```python
from build123d import *

# Parameters (mm, degrees)
SKETCH_1_W                   = 417.3
SKETCH_1_H                   = 60
EXTRUDE_1_DEPTH              = 23.5
SKETCH_2_W                   = 400
SKETCH_2_H                   = 45
CUT_EXTRUDE_1_DEPTH          = 10
SKETCH_3_W                   = 17.3
SKETCH_3_H                   = 60
EXTRUDE_2_DEPTH              = 19
HOLE_WIZARD_M3_1_D           = 2.5
HOLE_WIZARD_M3_1_DEPTH       = 7.5
HOLE_WIZARD_M3_1_CSINK_D     = 3.05
HOLE_WIZARD_M3_1_CSINK_ANGLE = 90
HOLE_WIZARD_M3_1_TIP         = 0.751075774
FILLET_1_R                   = 5
FILLET_2_R                   = 3
SKETCH_6_R                   = 13
CUT_EXTRUDE_2_DEPTH          = 20
HOLE_WIZARD_M4_1_D           = 3.3
HOLE_WIZARD_M4_1_DEPTH       = 10.1
HOLE_WIZARD_M4_1_CSINK_D     = 4.05
HOLE_WIZARD_M4_1_CSINK_ANGLE = 90
HOLE_WIZARD_M4_1_TIP         = 0.991420021
SKETCH_9_R                   = 2.25
CUT_EXTRUDE_3_DEPTH          = 15


with BuildPart() as part:
    # 草图1 → 凸台-拉伸1 (new body)
    with BuildSketch(Plane.XY):
        with Locations((208.65, -30)):
            Rectangle(SKETCH_1_W, SKETCH_1_H)
    extrude(amount=EXTRUDE_1_DEPTH)

    # 草图2 → 切除-拉伸1 (cut)
    with BuildSketch(Plane.XY.offset(23.5)):
        with Locations((217.3, -30)):
            Rectangle(SKETCH_2_W, SKETCH_2_H)
    extrude(amount=-CUT_EXTRUDE_1_DEPTH, mode=Mode.SUBTRACT)

    # 草图3 → 凸台-拉伸2 (add)
    with BuildSketch(Plane.XY.offset(23.5)):
        with Locations((8.65, -30)):
            Rectangle(SKETCH_3_W, SKETCH_3_H)
    extrude(amount=EXTRUDE_2_DEPTH)

    # M3 螺纹孔1
    with Locations(Plane(origin=(417.3, 0, 0), x_dir=(0, 0, -1), z_dir=(1, 0, 0))):
        with Locations((-4.75, -4), (-18.75, -4), (-18.75, -56), (-4.75, -56)):
            CounterSinkHole(HOLE_WIZARD_M3_1_D / 2, HOLE_WIZARD_M3_1_CSINK_D / 2, depth=HOLE_WIZARD_M3_1_DEPTH, counter_sink_angle=HOLE_WIZARD_M3_1_CSINK_ANGLE)
            with Locations((0, 0, -(HOLE_WIZARD_M3_1_DEPTH + HOLE_WIZARD_M3_1_TIP / 2))):  # 118° drill point
                Cone(0, HOLE_WIZARD_M3_1_D / 2, HOLE_WIZARD_M3_1_TIP, mode=Mode.SUBTRACT)

    # 圆角1
    fillet_1_edges = [part.edges().sort_by_distance(p)[0] for p in [
        (217.3, 0, 23.5),
        (217.3, -60, 23.5),
        (208.65, 0, 0),
        (208.65, -60, 0),
    ]]
    fillet(fillet_1_edges, radius=FILLET_1_R)

    # 圆角2
    fillet_2_edges = [part.edges().sort_by_distance(p)[0] for p in [
        (8.65, -60, 42.5),
        (8.65, 0, 42.5),
    ]]
    fillet(fillet_2_edges, radius=FILLET_2_R)

    # 草图6 → 切除-拉伸2 (cut)
    with BuildSketch(Plane.ZY):
        with Locations(Location((21.3, -30, 0), (0, 0, 270))):
            Circle(SKETCH_6_R)
    extrude(amount=-CUT_EXTRUDE_2_DEPTH, mode=Mode.SUBTRACT)

    # M4 螺纹孔1
    with Locations(Plane.ZY):
        with Locations((9.25, -11), (33.25, -11), (33.25, -49), (9.25, -49)):
            CounterSinkHole(HOLE_WIZARD_M4_1_D / 2, HOLE_WIZARD_M4_1_CSINK_D / 2, depth=HOLE_WIZARD_M4_1_DEPTH, counter_sink_angle=HOLE_WIZARD_M4_1_CSINK_ANGLE)
            with Locations((0, 0, -(HOLE_WIZARD_M4_1_DEPTH + HOLE_WIZARD_M4_1_TIP / 2))):  # 118° drill point
                Cone(0, HOLE_WIZARD_M4_1_D / 2, HOLE_WIZARD_M4_1_TIP, mode=Mode.SUBTRACT)

    # 草图9 → 切除-拉伸3 (cut)
    with BuildSketch(Plane(origin=(0, 0, 0), x_dir=(-1, 0, 0), z_dir=(0, 0, -1))):
        with Locations((-367.3, -15)):
            Circle(SKETCH_9_R)
        with Locations((-267.3, -15)):
            Circle(SKETCH_9_R)
        with Locations((-167.3, -15)):
            Circle(SKETCH_9_R)
        with Locations((-67.3, -15)):
            Circle(SKETCH_9_R)
        with Locations((-267.3, -45)):
            Circle(SKETCH_9_R)
        with Locations((-167.3, -45)):
            Circle(SKETCH_9_R)
        with Locations((-67.3, -45)):
            Circle(SKETCH_9_R)
        with Locations((-367.3, -45)):
            Circle(SKETCH_9_R)
    extrude(amount=-CUT_EXTRUDE_3_DEPTH, mode=Mode.SUBTRACT)


solid = part.part
```
Work out the finished part from the listing and answer in its coordinate system (mm). A direction names the side the tool comes from. Coordinates: 2 decimals unless noted, no trailing zeros. Write each loop counter-clockwise with the first axis right and the second up, starting at its lowest first coordinate (ties: lowest second). Pieces come first, ordered by that corner, then holes.
Q1. Which of the six approach directions +Z, -Z, +X, -X, +Y, -Y give full straight-line access (tool end or side, diameter ignored) to faces 1 (the face through (9.86, -27.18, 8.61)), 2 (the face through (215, -52.5, 19)), 3 (the face through (9, -30, 42.5))?
Q2. Each of these flat-tipped pins is pushed along its axis until it touches: pin 1 Ø3 at (x, y) = (257, -6) entering from +Z; pin 2 Ø2 at (y, z) = (-4, 18.75) entering from +X; pin 3 Ø12 at (x, y) = (199, -29) entering from +Z. Where does it stop, or does it pass through?
Q3. A cutting plane is placed at A-A, the plane y = -30. Give the vertices of the cut face in (x, z), then the cut area to 3 significant figures.
Q4. A cutting plane is placed at B-B, the plane x = 179. Give the vertices of the cut face in (y, z).
Q5. Find the intervals of material crossed by line 1 (Z direction, x = 4, y = -11); line 2 (Y direction, x = 306.5, z = 23); line 3 (Y direction, x = 7, z = 33.25), in increasing order.
Findings below:
1. face 1: -X
1. face 2: +Z, +X
1. face 3: +Z, +X, -X, +Y, -Y
2. pin 1: stops at z = 23.5
2. pin 2: stops at x = 409.65
2. pin 3: stops at z = 13.5
3. outline: (0, 0) - (417.3, 0) - (417.3, 13.5) - (20, 13.5) - (20, 8.3) - (0, 8.3) - close; (0, 34.3) - (17.3, 34.3) - (17.3, 42.5) - (0, 42.5) - close
3. area: 5,670 mm2
4. outline: (-60, 5) arc R5 ccw to (-55, 0) - (-5, 0) arc R5 ccw to (0, 5) - (0, 18.5) arc R5 ccw to (-5, 23.5) - (-7.5, 23.5) - (-7.5, 13.5) - (-52.5, 13.5) - (-52.5, 23.5) - (-55, 23.5) arc R5 ccw to (-60, 18.5) - close
5. line 1: z = 0 to 7.6, 10.9 to 31.6, 34.9 to 42.5
5. line 2: y = -57.18 to -52.5, -7.5 to -2.82
5. line 3: y = -60 to -50.65, -47.35 to -35.12, -24.88 to -12.65, -9.35 to 0
